Check sheet for the drawn part. Datum: minimum x, y, z corner. Units: mm. A direction names the side the tool comes from. Give positions to 0.01 mm unless a question says otherwise; leave off trailing zeros. Loops run counter-clockwise (first coordinate to the right, second up) from the corner with the lowest first, then second, coordinate; pieces in that order, holes last. Notation, with made-up numbers: (-31, -11) - (23, -11) arc R20 cw to (23, 17) - close; hole circle Ø7 at (85.5, -2.75). An arc over 180 degrees is marked (long way). Use one line per item in the form item = value.
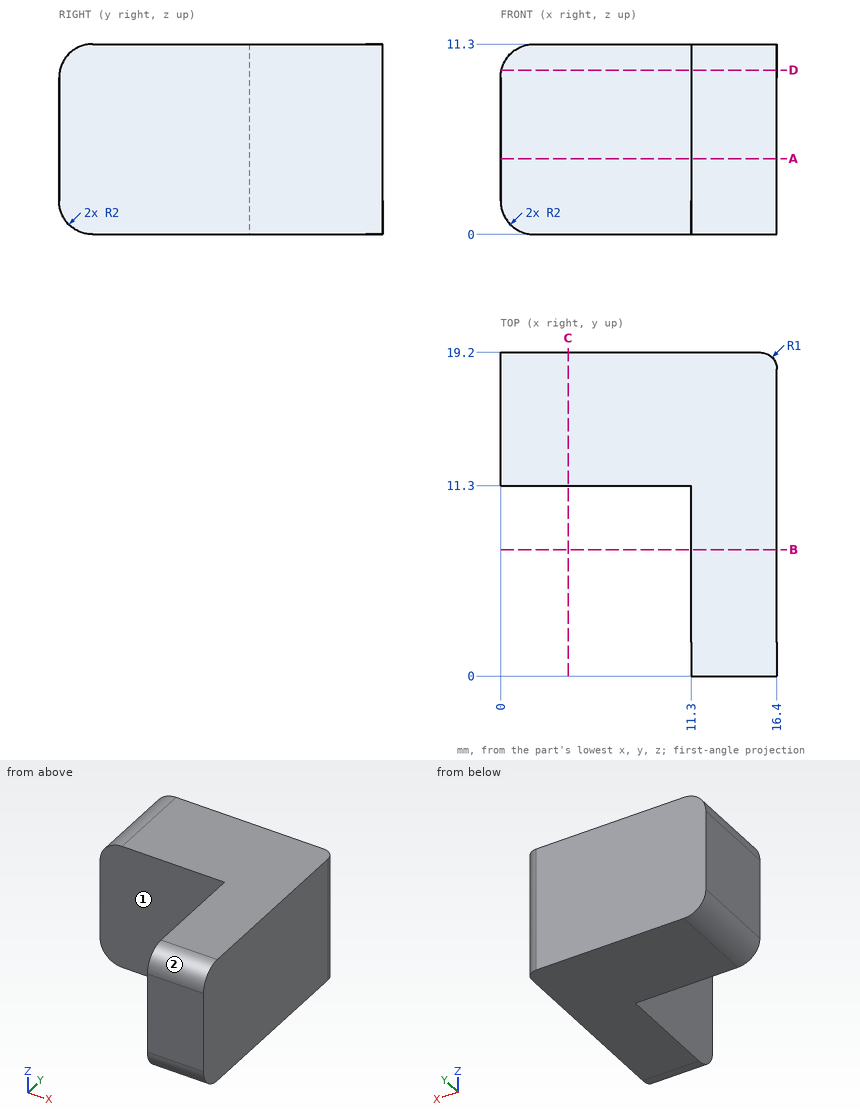
Item 1: Section check C-C on x = 4. Record the boundary of the cut face in (y, z).
Answer block:
outline = (11.3, 0) - (19.2, 0) - (19.2, 11.3) - (11.3, 11.3) - close
Item 2: Gauge pin test, flat end, axial feed: P1, Ø8, axis at x = 4, y = 5.5, coming from the +Z side. Record the tip position at first contact, or that the pin passes through.
Answer block:
P1 = through
Item 3: Section check D-D on z = 9.75. Record the boundary of the cut face in (x, y), then the cut area to 3 significant figures.
Answer block:
outline = (0.05, 11.3) - (11.3, 11.3) - (11.3, 0.05) - (16.4, 0.05) - (16.4, 18.2) arc R1 ccw to (15.4, 19.2) - (0.05, 19.2) - close
area = 186 mm2
Item 4: Section check B-B on y = 7.5. Record the boundary of the cut face in (x, z), then the cut area to 3 significant figures.
Answer block:
outline = (11.3, 0) - (16.4, 0) - (16.4, 11.3) - (11.3, 11.3) - close
area = 57.6 mm2
Item 5: Access from +Z, -Z, +X, -X, +Y, -Y to the whole of each face (thin tool, end or side, straight path). Record for the marked faces 1 and 2.
Answer block:
face_1 = +Z, -Z, -X, -Y
face_2 = +Z, +X, -X, -Y
Item 6: Section check A-A on z = 4.5. Record the boundary of the cut face in (x, y), then the cut area to 3 significant figures.
Answer block:
outline = (0, 11.3) - (11.3, 11.3) - (11.3, 0) - (16.4, 0) - (16.4, 18.2) arc R1 ccw to (15.4, 19.2) - (0, 19.2) - close
area = 187 mm2
Item 7: Thickness scan on L1, parallel to X at y = 3, z = 8; L2, parallel to Y at x = 4, z = 7.5; L3, parallel to Y at x = 11.75, z = 10.5. Record the ranges inside material, lowest first.
Answer block:
L1 = 11.3 to 16.4
L2 = 11.3 to 19.2
L3 = 0.4 to 19.2
